```python
from build123d import *

# Parameters (mm, degrees)
F0_R     = 1.55
F0_R_2   = 5
F0_R_3   = 6
F1_DEPTH = 2.4


with BuildPart() as f1:
    # F0 (on Front) → F1 (new body)
    with BuildSketch(Plane.XZ):
        with BuildLine():
            Line((-113.922411, -36.624175), (-112.515368, -36.601163))
            Line((-112.515368, -36.601163), (-45.969084, -36.601163))
            Line((-45.969084, -36.601163), (-1.763381, -39.740575))
            ThreePointArc((-1.763381, -39.740575), (14.757574, -26.757854), (2.545472, -9.659388))
            ThreePointArc((2.545472, -9.659388), (2.450522, -9.620676), (2.378003, -9.548185))
            Line((2.378003, -9.548185), (2.141578, -9.192446))
            ThreePointArc((2.141578, -9.192446), (1.519301, -7.870399), (1.305798, -6.424906))
            Line((1.305798, -6.424906), (1.305798, 23.520728))
            ThreePointArc((1.305798, 23.520728), (1.489272, 24.862771), (2.026229, 26.106321))
            Line((2.026229, 26.106321), (17.961467, 52.481679))
            ThreePointArc((17.961467, 52.481679), (18.021625, 56.515619), (14.537812, 58.550154))
            Line((14.537812, 58.550154), (-28.732704, 58.550154))
            Line((-28.732704, 58.550154), (-49.044828, 58.550154))
            ThreePointArc((-49.044828, 58.550154), (-50.662338, 58.208523), (-52.003552, 57.241984))
            Line((-52.003552, 57.241984), (-52.11812, 57.116057))
            ThreePointArc((-52.11812, 57.116057), (-53.794637, 55.907885), (-55.816525, 55.480845))
            Line((-55.816525, 55.480845), (-61.90531, 55.480845))
            ThreePointArc((-61.90531, 55.480845), (-62.687482, 55.542404), (-63.450395, 55.725563))
            Line((-63.450395, 55.725563), (-72.478836, 58.659081))
            Line((-72.478836, 58.659081), (-122.961926, 75.062031))
            ThreePointArc((-122.961926, 75.062031), (-126.776963, 74.761781), (-129.262293, 71.851834))
            Line((-129.262293, 71.851834), (-129.57131, 70.900777))
            Line((-129.57131, 70.900777), (-74.332938, 52.952742))
            Line((-74.332938, 52.952742), (-68.495444, 51.056025))
            Line((-68.495444, 51.056025), (-62.997354, 49.269588))
            Line((-62.997354, 49.269588), (-70.440539, 26.36182))
            Line((-70.440539, 26.36182), (-75.938629, 28.148258))
            Line((-75.938629, 28.148258), (-81.749346, 30.127386))
            Line((-81.749346, 30.127386), (-115.36281, 41.049062))
            Line((-115.36281, 41.049062), (-136.987718, 48.075421))
            Line((-136.987718, 48.075421), (-137.296735, 47.124364))
            ThreePointArc((-137.296735, 47.124364), (-137.251084, 43.900182), (-135.246711, 41.374332))
            ThreePointArc((-135.246711, 41.374332), (-134.684364, 41.061766), (-134.086537, 40.823997))
            Line((-134.086537, 40.823997), (-72.970283, 20.966122))
            ThreePointArc((-72.970283, 20.966122), (-70.470283, 19.149766), (-69.515368, 16.210839))
            Line((-69.515368, 16.210839), (-69.515368, -9.553598))
            ThreePointArc((-69.515368, -9.553598), (-70.101155, -10.967812), (-71.515368, -11.553598))
            Line((-71.515368, -11.553598), (-74.523215, -11.553598))
            Line((-74.523215, -11.553598), (-112.515368, -11.553598))
            ThreePointArc((-112.515368, -11.553598), (-112.528511, -11.553641), (-112.541654, -11.553771))
            Line((-112.541654, -11.553771), (-114.961689, -11.569675))
            ThreePointArc((-114.961689, -11.569675), (-115.664544, -11.864874), (-115.955117, -12.569653))
            Line((-115.955117, -12.569653), (-115.955117, -34.624443))
            ThreePointArc((-115.955117, -34.624443), (-115.35772, -36.050173), (-113.922411, -36.624175))
        make_face()
        with Locations((-112.955117, -33.601163)):
            Circle(F0_R, mode=Mode.SUBTRACT)
        with Locations((-112.955117, -17.601163)):
            Circle(F0_R, mode=Mode.SUBTRACT)
        with Locations((-64.515368, -6.553598)):
            Circle(F0_R, mode=Mode.SUBTRACT)
        with Locations((-64.515368, 14.843552)):
            Circle(F0_R, mode=Mode.SUBTRACT)
        with Locations((-10.015368, -35.974115)):
            Circle(F0_R, mode=Mode.SUBTRACT)
        with Locations((-0.298833, -33.601163)):
            Circle(F0_R, mode=Mode.SUBTRACT)
        with Locations((-18.015368, -20.601163)):
            Circle(F0_R_2, mode=Mode.SUBTRACT)
        with Locations((-9.298833, -24.601163)):
            Circle(F0_R, mode=Mode.SUBTRACT)
        with Locations((-0.298833, -24.601163)):
            Circle(F0_R_3, mode=Mode.SUBTRACT)
        with Locations((8.701167, -24.601163)):
            Circle(F0_R, mode=Mode.SUBTRACT)
        with Locations((-0.298833, -15.601163)):
            Circle(F0_R, mode=Mode.SUBTRACT)
        with Locations((-21.515368, -6.553598)):
            Circle(F0_R, mode=Mode.SUBTRACT)
        with BuildLine():
            Line((-26.515368, -11.553598), (-57.515368, -11.553598))
            ThreePointArc((-57.515368, -11.553598), (-58.929582, -10.967812), (-59.515368, -9.553598))
            Line((-59.515368, -9.553598), (-59.515368, 17.843552))
            ThreePointArc((-59.515368, 17.843552), (-58.929582, 19.257766), (-57.515368, 19.843552))
            Line((-57.515368, 19.843552), (-26.515368, 19.843552))
            ThreePointArc((-26.515368, 19.843552), (-25.390432, 19.49719), (-24.655131, 18.57807))
            ThreePointArc((-24.655131, 18.57807), (-24.55062, 18.2174), (-24.515368, 17.843552))
            Line((-24.515368, 17.843552), (-24.515368, -9.553598))
            ThreePointArc((-24.515368, -9.553598), (-24.55062, -9.927447), (-24.655131, -10.288116))
            ThreePointArc((-24.655131, -10.288116), (-25.390432, -11.207236), (-26.515368, -11.553598))
        make_face(mode=Mode.SUBTRACT)
        with Locations((-21.515368, 14.843552)):
            Circle(F0_R, mode=Mode.SUBTRACT)
        with BuildLine():
            ThreePointArc((-9.597609, 7.890928), (-6.738423, 7.027389), (-4.649818, 4.892354))
            Line((-4.649818, 4.892354), (-4.649818, -1.10003))
            ThreePointArc((-4.649818, -1.10003), (-4.685937, -1.161841), (-4.722791, -1.223217))
            ThreePointArc((-4.722791, -1.223217), (-7.08024, -3.427238), (-10.238487, -4.091129))
            ThreePointArc((-10.238487, -4.091129), (-15.82221, 0.503221), (-12.932287, 7.13152))
            ThreePointArc((-12.932287, 7.13152), (-11.320202, 7.753855), (-9.597609, 7.890928))
        make_face(mode=Mode.SUBTRACT)
        with Locations((-38.631012, 31.451518)):
            Circle(F0_R, mode=Mode.SUBTRACT)
        with Locations((-44.512843, 32.636452)):
            Circle(F0_R, mode=Mode.SUBTRACT)
        with Locations((-43.13741, 38.056231)):
            Circle(F0_R, mode=Mode.SUBTRACT)
        with Locations((-41.23285, 43.326407)):
            Circle(F0_R, mode=Mode.SUBTRACT)
        with Locations((-37.400858, 36.297828)):
            Circle(F0_R, mode=Mode.SUBTRACT)
        with Locations((-35.702059, 41.000389)):
            Circle(F0_R, mode=Mode.SUBTRACT)
        with BuildLine():
            Line((-23.838282, 52.000154), (-45.838282, 52.000154))
            ThreePointArc((-45.838282, 52.000154), (-47.388282, 53.550154), (-45.838282, 55.100154))
            Line((-45.838282, 55.100154), (-23.838282, 55.100154))
            ThreePointArc((-23.838282, 55.100154), (-22.288282, 53.550154), (-23.838282, 52.000154))
        make_face(mode=Mode.SUBTRACT)
        with BuildLine():
            Line((9.161718, 52.000154), (-12.838282, 52.000154))
            ThreePointArc((-12.838282, 52.000154), (-14.388282, 53.550154), (-12.838282, 55.100154))
            Line((-12.838282, 55.100154), (9.161718, 55.100154))
            ThreePointArc((9.161718, 55.100154), (10.711718, 53.550154), (9.161718, 52.000154))
        make_face(mode=Mode.SUBTRACT)
        Polygon((-129.57131, 70.900777), (-136.987718, 48.075421), (-115.36281, 41.049062), (-81.749346, 30.127386), (-75.938629, 28.148258), (-70.440539, 26.36182), (-62.997354, 49.269588), (-68.495444, 51.056025), (-74.332938, 52.952742), align=None)
        with Locations((-73.650736, 32.662188)):
            Circle(F0_R, mode=Mode.SUBTRACT)
        with Locations((-69.297722, 46.05939)):
            Circle(F0_R, mode=Mode.SUBTRACT)
        with Locations((-130.68735, 51.285618)):
            Circle(F0_R, mode=Mode.SUBTRACT)
        with Locations((-126.361112, 64.60041)):
            Circle(F0_R, mode=Mode.SUBTRACT)
    extrude(amount=F1_DEPTH)


solid = f1.part
```
Work out the finished part from the listing and answer in its coordinate system (mm). A direction names the side the tool comes from. Round coordinates to 2 decimals unless told otherwise and drop trailing zeros. Loops run counter-clockwise (first coordinate to the right, second up) from the corner with the lowest first, then second, coordinate; pieces in that order, holes last. Notation, with made-up numbers: M -26,67.5 L 1,67.5 A18 cw 1,94.5 Z; hole C 87,7 d2. An arc over 180 degrees is marked long. Use CSV: the item, a comma, the result in double quotes.
Q1. The mould has two halves that part along X. Classify faces 3 (the flat face through (-24.18, -1.18, -38.15)), 4 (the cylindrical face through (-72.936, -1.183, 31.287)), 5 (the flat face through (-61, -2.4, 19)), 6 (the cylindrical face through (-0.501, -1.183, -14.064)): pulls with the +X half, pulls with the -X half, needs draft (parallel to the pull), parting line crosses it, or undercut.
Determined:
face 3,"pulls with the -X half"
face 4,"undercut"
face 5,"needs draft"
face 6,"undercut"
Q2. A tool of negligible diameter and unlimited length cuts with its end or side. For faces 1 (the cylindrical face through (-1.6, -1.18, -30.46)), 2 (the cylindrical face through (-70.5, -1.18, 19.19)), from which of +Z, -Z, +X, -X, +Y, -Y can it reach the whole face along a straight path? Write none if from no direction.
Determined:
face 1,"+Y, -Y"
face 2,"-X, +Y, -Y"
Q3. Each of these flat-tipped pins is pushed along its axis until it touches: pin 1 (3.5 mm diameter, centred on x = -44.51, z = 32.64, fed in from +Y); pin 2 (0.7 mm diameter, centred on x = -0.5, y = -0.5, fed in from +Z); pin 3 (1.2 mm diameter, centred on y = -1.5, z = 8.5, fed in from -X). Where does it stop, or does it pass through?
Determined:
pin 1,"y = 0"
pin 2,"z = 58.55"
pin 3,"x = -69.52"
Q4. Section D-D, the plane y = -1.6 is taken. State how many separate pieces and enclosed holes the cut face has, then the cut area to 3 significant figures.
Determined:
separate pieces,"1"
enclosed holes,"27"
area,"9,280 mm2"
Q5. Consider L1, parallel to X at y = -2, z = 8; L2, parallel to X at y = -0.3, z = -2; L3, parallel to Z at x = -7, y = -1.55. Determine where each line is inside the solid, lowest interval first.
Determined:
L1,"-69.52 to -59.52, -24.52 to 1.31"
L2,"-69.52 to -59.52, -24.52 to -14.54, -5.29 to 1.31"
L3,"-39.37 to -3.38, 7.18 to 52, 55.1 to 58.55"
Q6. Section C-C, the plane z = -28 is taken. Determine the outline of the cut face in (x, y).
Determined:
outline,"M -115.96,-2.4 L -5.24,-2.4 L -5.24,0 L -115.96,0 Z; M 4.65,-2.4 L 14.53,-2.4 L 14.53,0 L 4.65,0 Z"
Q7. Section A-A, the plane x = -109 is taken. Determine the outline of the cut face in (y, z), then the cut area to 3 significant figures.
Determined:
outline,"M -2.4,-36.6 L 0,-36.6 L 0,-11.55 L -2.4,-11.55 Z; M -2.4,32.67 L 0,32.67 L 0,70.53 L -2.4,70.53 Z"
area,"151 mm2"
Q8. Section B-B, the plane x = -31.5 is taken. Determine the outline of the cut face in (y, z).
Determined:
outline,"M -2.4,-37.63 L 0,-37.63 L 0,-11.55 L -2.4,-11.55 Z; M -2.4,19.84 L 0,19.84 L 0,52 L -2.4,52 Z; M -2.4,55.1 L 0,55.1 L 0,58.55 L -2.4,58.55 Z"
